Model file for the job. Use its own axes, mm. A direction names the side the tool comes from. Round coordinates to 2 decimals unless told otherwise and drop trailing zeros. Order: outer loops, then holes, each group sorted by start corner. A loop starts at its lowest first (then second) coordinate and runs counter-clockwise, first axis right, second up. Notation, with made-up numbers: (69.5, 74.25) - (102.5, 74.25) arc R14 ccw to (102.5, 82.25) - close; hole circle Ø4 at (9, 3). An arc over 180 degrees is marked (long way). Write item = value, one per line.
```python
from build123d import *

# Parameters (mm, degrees)
F1_DEPTH      = 1
F3_DEPTH      = 27
F5_DEPTH      = 1
F7_DEPTH      = 13
F8_R          = 1.5
F9_DEPTH      = 25
F10_DEPTH     = 5
F11_T1_DEPTH  = 29
F11_T3_DEPTH  = 13
F11_T5_DEPTH  = 27
F11_T7_DEPTH  = 30.5
F11_T9_DEPTH  = 30.5
F11_T11_DEPTH = 53.0467878714
F11_T13_DEPTH = 27


# Not quite as in the source:
# - a fillet or chamfer that OpenCascade refuses, or shapes differently, is made with other operations: its cross-section is extruded or revolved along the edge and cut away or added


with BuildPart() as f1:
    # F0 (on Top) → F1 (new body)
    with BuildSketch(Plane.XY):
        Polygon((0, 34.9576839236), (0, 0), (47.9637535727, -1.8650316928), (48.9898140027, 0.9540461696), (27, 8.9576839236), (27, 34.9576839236), align=None)
    extrude(amount=F1_DEPTH)

    # F2 (on face) → F3 (join)
    with BuildSketch(Plane.XY.offset(1)):
        Polygon((2.5, 34.9576839236), (0, 34.9576839236), (0, 0), (47.9637535727, -1.8650316928), (48.1792508796, -1.2729577082), (2.5, 0.5032429485), align=None)
        Polygon((27, 34.9576839236), (19, 34.9576839236), (19, 11.2309391343), (48.7846019167, 0.3902305971), (48.9898140027, 0.9540461696), (27, 8.9576839236), align=None)
    extrude(amount=F3_DEPTH)

    # F4 (on face) → F5 (join)
    with BuildSketch(Plane.XY.offset(28)):
        Polygon((0, 34.9576839236), (0, 0), (47.9637535727, -1.8650316928), (48.9898140027, 0.9540461696), (27, 8.9576839236), (27, 34.9576839236), align=None)
    extrude(amount=F5_DEPTH)

    # F6 (on face) → F7 (join)
    with BuildSketch(Plane(origin=(0, 0, 0), x_dir=(1, 0, 0), z_dir=(0, 0, -1))):
        Polygon((27, -64.9576839236), (27, -34.9576839236), (19, -34.9576839236), (19, -75.9576839236), (24.5, -75.9576839236), (24.5, -64.9576839236), align=None)
    extrude(amount=-F7_DEPTH)

    # F8 (on face) → F9 (cut)
    with BuildSketch(Plane(origin=(19, 0, 0), x_dir=(0, -1, 0), z_dir=(-1, 0, 0))):
        with Locations((-72.9576839236, 4.5)):
            Circle(F8_R)
        with BuildLine():
            Line((-32.8452885151, 11), (-57.2458393872, 11))
            ThreePointArc((-57.2458393872, 11), (-58.9458393872, 9.3), (-57.2458393872, 7.6))
            Line((-57.2458393872, 7.6), (-32.8452885151, 7.6))
            ThreePointArc((-32.8452885151, 7.6), (-31.1452885151, 9.3), (-32.8452885151, 11))
        make_face()
    extrude(amount=-F9_DEPTH, mode=Mode.SUBTRACT)

    # F8 (on face) → F10 (cut)
    with BuildSketch(Plane(origin=(19, 0, 0), x_dir=(0, -1, 0), z_dir=(-1, 0, 0))):
        with BuildLine():
            Line((-32.8452885151, 12.3), (-57.2458393872, 12.3))
            ThreePointArc((-57.2458393872, 12.3), (-60.2458393872, 9.3), (-57.2458393872, 6.3))
            Line((-57.2458393872, 6.3), (-32.8452885151, 6.3))
            ThreePointArc((-32.8452885151, 6.3), (-29.8452885151, 9.3), (-32.8452885151, 12.3))
        make_face()
        with BuildLine():
            ThreePointArc((-57.2458393872, 7.6), (-58.9458393872, 9.3), (-57.2458393872, 11))
            Line((-57.2458393872, 11), (-32.8452885151, 11))
            ThreePointArc((-32.8452885151, 11), (-31.1452885151, 9.3), (-32.8452885151, 7.6))
            Line((-32.8452885151, 7.6), (-57.2458393872, 7.6))
        make_face(mode=Mode.SUBTRACT)
    extrude(amount=-F10_DEPTH, mode=Mode.SUBTRACT)

    # F11: fillet of radius 5 on 7 edges, made by hand

    # F11_s2 → F11_t1 (join)
    with BuildSketch(Plane.XY):
        with BuildLine():
            ThreePointArc((27, 12.4587216147), (27.9042397786, 9.5908394329), (30.2898992834, 7.7602585108))
            Line((30.2898992834, 7.7602585108), (27, 8.9576839236))
            Line((27, 8.9576839236), (27, 12.4587216147))
        make_face()
    extrude(amount=F11_T1_DEPTH)

    # F11_s4 → F11_t3 (join)
    with BuildSketch(Plane.XY):
        with BuildLine():
            ThreePointArc((27, 64.9576839236), (25.1698729811, 66.7878109426), (24.5, 69.2878109426))
            Line((24.5, 69.2878109426), (24.5, 64.9576839236))
            Line((24.5, 64.9576839236), (27, 64.9576839236))
        make_face()
    extrude(amount=F11_T3_DEPTH)

    # F11_s6 → F11_t5 (join)
    with BuildSketch(Plane.XY.offset(1)):
        with BuildLine():
            ThreePointArc((2.5, 5.3126005228), (3.8964343579, 1.8464333797), (7.3057258653, 0.3163761923))
            Line((7.3057258653, 0.3163761923), (2.5, 0.5032429485))
            Line((2.5, 0.5032429485), (2.5, 5.3126005228))
        make_face()
    extrude(amount=F11_T5_DEPTH)

    # F11_s8 → F11_t7 (cut)
    with BuildSketch(Plane.YZ.offset(6.5)):
        with BuildLine():
            ThreePointArc((70.9576839236, 0), (74.4932178296, 1.4644660941), (75.9576839236, 5))
            Line((75.9576839236, 5), (75.9576839236, 0))
            Line((75.9576839236, 0), (70.9576839236, 0))
        make_face()
    extrude(amount=F11_T7_DEPTH, mode=Mode.SUBTRACT)

    # F11_s10 → F11_t9 (cut)
    with BuildSketch(Plane.YZ.offset(6.5)):
        with BuildLine():
            ThreePointArc((70.9576839236, 13), (74.4932178296, 11.5355339059), (75.9576839236, 8))
            Line((75.9576839236, 8), (75.9576839236, 13))
            Line((75.9576839236, 13), (70.9576839236, 13))
        make_face()
    extrude(amount=F11_T9_DEPTH, mode=Mode.SUBTRACT)

    # F11_s12 → F11_t11 (cut)
    with BuildSketch(Plane.XY.offset(-12.0233939357)):
        with BuildLine():
            ThreePointArc((4.8057258653, -0.1868667562), (1.3964343579, 1.3431904313), (0, 4.8093575743))
            Line((0, 4.8093575743), (0, 0))
            Line((0, 0), (4.8057258653, -0.1868667562))
        make_face()
    extrude(amount=F11_T11_DEPTH, mode=Mode.SUBTRACT)

    # F11_s14 → F11_t13 (cut)
    with BuildSketch(Plane.XY.offset(1)):
        with BuildLine():
            ThreePointArc((19, 14.7319768253), (19.9042397786, 11.8640946436), (22.2898992834, 10.0335137214))
            Line((22.2898992834, 10.0335137214), (19, 11.2309391343))
            Line((19, 11.2309391343), (19, 14.7319768253))
        make_face()
    extrude(amount=F11_T13_DEPTH, mode=Mode.SUBTRACT)


solid = f1.part
```
1) Mould opens along X. For faces 4 (the face through (35.35, 5.28, 14.31)), 5 (the face through (25.479, 31.146, 9.263)), 6 (the face through (25.188, 66.756, 6.409)) say: +X half, -X half, draft (parallel to the pull), parting line (faces both ways), or undercut.
Conclusion:
face_4 = undercut
face_5 = draft
face_6 = +X half
2) Flat gauge pins, fed straight in: pin 1 Ø8 at (x, y) = (26, 12.5) entering from -Z; pin 2 Ø3 at (x, z) = (7.5, 16) entering from -Y; pin 3 Ø6.5 at (x, y) = (21.5, 47.5) entering from +Z; pin 4 Ø14 at (y, z) = (52.5, 15.5) entering from -X. Where does each tip first touch, or does it go through?
Conclusion:
pin_1 = 0
pin_2 = -0.35
pin_3 = 13
pin_4 = 19
3) 3-axis set-ups, long thin cutter, end or side, ignore diameter. For faces 1 (the face through (23, 53, 13)), 2 (the face through (21.465, 29.846, 9.234)), 3 (the face through (21.465, 60.245, 9.366)): which of +Z, -Z, +X, -X, +Y, -Y reach the whole face in a straight line?
Conclusion:
face_1 = +Z, +X, -X, +Y
face_2 = none
face_3 = -X
4) Cut at C-C (x = 33). Write the cut outline in (y, z), and give its area (3 significant figures).
Conclusion:
outline = (-1.28, 0) - (6.77, 0) - (6.77, 29) - (-1.28, 29) - close; hole (-0.68, 1) - (6.14, 1) - (6.14, 28) - (-0.68, 28) - close
area = 49.6 mm^2
5) Cut at D-D (z = 9.3). Write the cut outline in (x, y), and give its area (3 significant figures).
Conclusion:
outline = (0, 4.81) arc R5 ccw to (4.81, -0.19) - (47.96, -1.87) - (48.18, -1.27) - (7.31, 0.32) arc R5 cw to (2.5, 5.31) - (2.5, 34.96) - (0, 34.96) - close; (19, 14.73) arc R5 ccw to (22.29, 10.03) - (48.78, 0.39) - (48.99, 0.95) - (30.29, 7.76) arc R5 cw to (27, 12.46) - (27, 31.15) - (24, 31.15) - (24, 29.85) - (19, 29.85) - close; (19, 60.25) - (24, 60.25) - (24, 58.95) - (27, 58.95) - (27, 64.96) arc R5 cw to (24.5, 69.29) - (24.5, 75.79) - (19, 75.79) - close
area = 398 mm^2
6) Cut at B-B (z = 16.5). Write the cut outline in (x, y), and give its area (3 significant figures).
Conclusion:
outline = (0, 4.81) arc R5 ccw to (4.81, -0.19) - (47.96, -1.87) - (48.18, -1.27) - (7.31, 0.32) arc R5 cw to (2.5, 5.31) - (2.5, 34.96) - (0, 34.96) - close; (19, 14.73) arc R5 ccw to (22.29, 10.03) - (48.78, 0.39) - (48.99, 0.95) - (30.29, 7.76) arc R5 cw to (27, 12.46) - (27, 34.96) - (19, 34.96) - close
area = 330 mm^2
7) Wall check: line 1 along Z through (x, y) = (22.5, 41); line 2 along X through (y, z) = (21.5, 5.5); line 3 along Z through (x, y) = (19.5, 34). Give the ranges that are in metal, low to high.
Conclusion:
line_1 = 0 to 6.3, 12.3 to 13
line_2 = 0 to 2.5, 19 to 27
line_3 = 0 to 6.3, 12.3 to 29
8) Cut at A-A (y = 51). Write the cut outline in (x, z).
Conclusion:
outline = (19, 0) - (27, 0) - (27, 7.6) - (24, 7.6) - (24, 6.3) - (19, 6.3) - close; (19, 12.3) - (24, 12.3) - (24, 11) - (27, 11) - (27, 13) - (19, 13) - close
